Can you work these out from the drawing? Everything is in mm from the part's minimum corner. A direction names the side the tool comes from. Coordinates: 2 decimals unless noted, no trailing zeros. Loops run counter-clockwise (first coordinate to the right, second up) from the corner with the lowest first, then second, coordinate; pieces in that order, holes last. Notation, with made-up numbers: (84.5, 29.5) -> (90.5, 29.5) arc R20 cw to (90.5, 47.5) -> close; hole circle Ø11 at (-8.75, 70.5). An arc over 180 degrees is marked (long way). Put each result on its own line as item: value. Start each with the question number.
Item 1: If we section it at D-D on z = 18.5: Please give me the cut outline in (x, y), plus the area to 3 significant figures.
Item 2: Will these pins go through, and if not, where does the flat tip stop? P1, Ø7, axis at x = 18, z = 13.5, coming from the +Y side; P2, Ø2, axis at y = 6, z = 26.5, coming from the +X side; P3, Ø5, axis at y = 14, z = 15.5, coming from the +X side; P4, Ø4.5, axis at x = 20, z = 10, coming from the +Y side.
Item 3: Please list where these lines run through material, in increasing order: L1, parallel to Z at x = 2.85, y = 20; L2, parallel to X at y = 31, z = 31.5. Write a range as from..to.
Item 4: We'd pull the mould along X, two halves only. Please class the marked faces 3, 4, 5 and 6: pulls with the +X half, pulls with the -X half, needs draft (parallel to the pull), parting line crosses it, or undercut.
Item 5: For the marked faces 1 and 2, which set-ups out of +Z, -Z, +X, -X, +Y, -Y let a thin tool reach every point of the face, with its end or its side?
Item 6: If we section it at A-A on z = 30: Please give me the cut outline in (x, y), plus the area to 3 significant figures.
Item 7: If we section it at B-B on x = 20: Please give me the cut outline in (y, z).
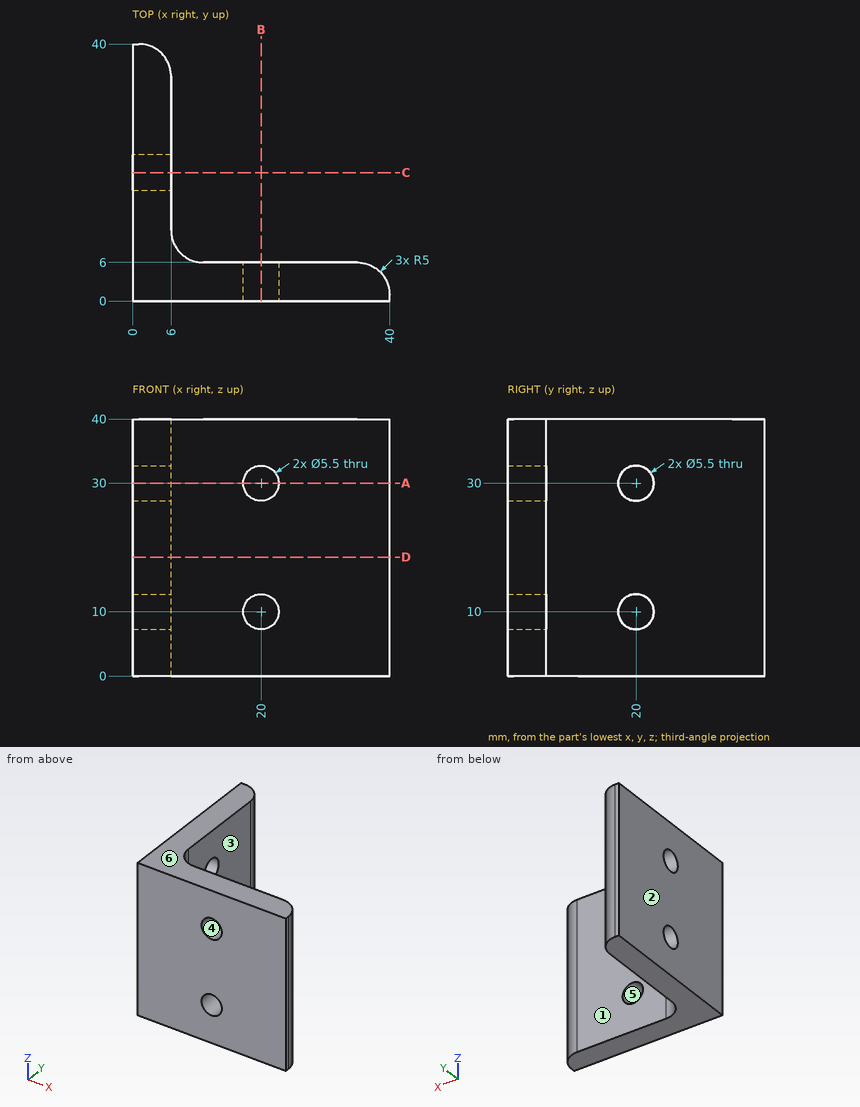
Solutions:
1. outline: (0, 0) -> (40, 0) -> (40, 1) arc R5 ccw to (35, 6) -> (11, 6) arc R5 cw to (6, 11) -> (6, 35) arc R5 ccw to (1, 40) -> (0, 40) -> close
1. area: 439 mm^2
2. P1: y = 6
2. P2: x = 38
2. P3: x = 6
2. P4: through
3. L1: 0..7.25, 12.75..27.25, 32.75..40
3. L2: 0..6
4. face 3: pulls with the +X half
4. face 4: undercut
4. face 5: undercut
4. face 6: needs draft
5. face 1: +Z, -Z, +X, +Y
5. face 2: +Z, -Z, -X, +Y, -Y
6. outline: (0, 0) -> (17.25, 0) -> (17.25, 6) -> (11, 6) arc R5 cw to (6, 11) -> (6, 17.25) -> (0, 17.25) -> close; (0, 22.75) -> (6, 22.75) -> (6, 35) arc R5 ccw to (1, 40) -> (0, 40) -> close; (22.75, 0) -> (40, 0) -> (40, 1) arc R5 ccw to (35, 6) -> (22.75, 6) -> close
6. area: 373 mm^2
7. outline: (0, 0) -> (6, 0) -> (6, 7.25) -> (0, 7.25) -> close; (0, 12.75) -> (6, 12.75) -> (6, 27.25) -> (0, 27.25) -> close; (0, 32.75) -> (6, 32.75) -> (6, 40) -> (0, 40) -> close
